from build123d import *

# Parameters (mm, degrees)
F0_R     = 10.002614
F0_W     = 8.257874
F0_H     = 10.88538
F0_R_2   = 19.05
F1_DEPTH = 3.175


with BuildPart() as f1:
    # F0 (on Front) → F1 (new body)
    with BuildSketch(Plane.XZ):
        with BuildLine():
            ThreePointArc((75.042351, -13.231991), (75.910036, -6.641268), (76.2, 0))
            ThreePointArc((76.2, 0), (76.134965, 3.14755), (75.939972, 6.289727))
            ThreePointArc((75.939972, 6.289727), (75.570922, 9.771172), (75.042351, 13.231991))
            ThreePointArc((75.042351, 13.231991), (72.726083, 22.745479), (69.209018, 31.88341))
            ThreePointArc((69.209018, 31.88341), (67.6715, 35.028675), (65.991136, 38.1))
            ThreePointArc((65.991136, 38.1), (60.560752, 46.247544), (54.130435, 53.631483))
            ThreePointArc((54.130435, 53.631483), (51.609896, 56.061204), (48.980416, 58.372587))
            ThreePointArc((48.980416, 58.372587), (41.0909, 64.171473), (32.522923, 68.910808))
            ThreePointArc((32.522923, 68.910808), (29.323378, 70.331924), (26.061935, 71.604578))
            ThreePointArc((26.061935, 71.604578), (16.664879, 74.355375), (6.992666, 75.878473))
            ThreePointArc((6.992666, 75.878473), (3.500027, 76.119576), (0, 76.2))
            ThreePointArc((0, 76.2), (-9.771172, 75.570922), (-19.381009, 73.694074))
            ThreePointArc((-19.381009, 73.694074), (-22.745479, 72.726083), (-26.061935, 71.604578))
            ThreePointArc((-26.061935, 71.604578), (-35.028675, 67.6715), (-43.417049, 62.621082))
            ThreePointArc((-43.417049, 62.621082), (-46.247544, 60.560752), (-48.980416, 58.372587))
            ThreePointArc((-48.980416, 58.372587), (-56.061204, 51.609896), (-62.216352, 43.995063))
            ThreePointArc((-62.216352, 43.995063), (-64.171473, 41.0909), (-65.991136, 38.1))
            ThreePointArc((-65.991136, 38.1), (-70.331924, 29.323378), (-73.511444, 20.06259))
            ThreePointArc((-73.511444, 20.06259), (-74.355375, 16.664879), (-75.042351, 13.231991))
            ThreePointArc((-75.042351, 13.231991), (-76.119576, 3.500027), (-75.939972, -6.289727))
            ThreePointArc((-75.939972, -6.289727), (-75.570922, -9.771172), (-75.042351, -13.231991))
            ThreePointArc((-75.042351, -13.231991), (-72.726083, -22.745479), (-69.209018, -31.88341))
            ThreePointArc((-69.209018, -31.88341), (-67.6715, -35.028675), (-65.991136, -38.1))
            ThreePointArc((-65.991136, -38.1), (-60.560752, -46.247544), (-54.130435, -53.631483))
            ThreePointArc((-54.130435, -53.631483), (-51.609896, -56.061204), (-48.980416, -58.372587))
            ThreePointArc((-48.980416, -58.372587), (-41.0909, -64.171473), (-32.522923, -68.910808))
            ThreePointArc((-32.522923, -68.910808), (-29.323378, -70.331924), (-26.061935, -71.604578))
            ThreePointArc((-26.061935, -71.604578), (-16.664879, -74.355375), (-6.992666, -75.878473))
            ThreePointArc((-6.992666, -75.878473), (-3.500027, -76.119576), (0, -76.2))
            ThreePointArc((0, -76.2), (9.771172, -75.570922), (19.381009, -73.694074))
            ThreePointArc((19.381009, -73.694074), (22.745479, -72.726083), (26.061935, -71.604578))
            ThreePointArc((26.061935, -71.604578), (35.028675, -67.6715), (43.417049, -62.621082))
            ThreePointArc((43.417049, -62.621082), (46.247544, -60.560752), (48.980416, -58.372587))
            ThreePointArc((48.980416, -58.372587), (56.061204, -51.609896), (62.216352, -43.995063))
            ThreePointArc((62.216352, -43.995063), (64.171473, -41.0909), (65.991136, -38.1))
            ThreePointArc((65.991136, -38.1), (70.331924, -29.323378), (73.511444, -20.06259))
            ThreePointArc((73.511444, -20.06259), (74.355375, -16.664879), (75.042351, -13.231991))
        make_face()
        with Locations((-32.771484, -33.103804)):
            Circle(F0_R, mode=Mode.SUBTRACT)
        with Locations((1.650614, -45.994491)):
            Circle(F0_R, mode=Mode.SUBTRACT)
        with Locations((35.105805, -30.769484)):
            Circle(F0_R, mode=Mode.SUBTRACT)
        with Locations((-47.996491, 0.351386)):
            Circle(F0_R, mode=Mode.SUBTRACT)
        with Locations((-25.4, 0)):
            Rectangle(F0_W, F0_H, mode=Mode.SUBTRACT)
        with Locations((-35.105805, 34.773484)):
            Circle(F0_R, mode=Mode.SUBTRACT)
        with Locations((-1.650614, 49.998491)):
            Circle(F0_R, mode=Mode.SUBTRACT)
        Circle(F0_R_2, mode=Mode.SUBTRACT)
        with Locations((25.4, 0)):
            Rectangle(F0_W, F0_H, mode=Mode.SUBTRACT)
        with Locations((32.771484, 37.107805)):
            Circle(F0_R, mode=Mode.SUBTRACT)
        with Locations((47.996491, 3.652614)):
            Circle(F0_R, mode=Mode.SUBTRACT)
        with BuildLine():
            ThreePointArc((75.042351, 13.231991), (75.570922, 9.771172), (75.939972, 6.289727))
            Line((75.939972, 6.289727), (93.646024, 16.512321))
            Line((93.646024, 16.512321), (75.042351, 13.231991))
        make_face()
        with BuildLine():
            Line((93.646024, -16.512321), (75.042351, -13.231991))
            ThreePointArc((75.042351, -13.231991), (74.355375, -16.664879), (73.511444, -20.06259))
            Line((73.511444, -20.06259), (93.646024, -16.512321))
        make_face()
        with BuildLine():
            ThreePointArc((65.991136, 38.1), (67.6715, 35.028675), (69.209018, 31.88341))
            Line((69.209018, 31.88341), (82.350931, 47.545332))
            Line((82.350931, 47.545332), (65.991136, 38.1))
        make_face()
        with BuildLine():
            Line((82.350931, -47.545332), (65.991136, -38.1))
            ThreePointArc((65.991136, -38.1), (64.171473, -41.0909), (62.216352, -43.995063))
            Line((62.216352, -43.995063), (82.350931, -47.545332))
        make_face()
        with BuildLine():
            ThreePointArc((48.980416, 58.372587), (51.609896, 56.061204), (54.130435, 53.631483))
            Line((54.130435, 53.631483), (61.123101, 72.843675))
            Line((61.123101, 72.843675), (48.980416, 58.372587))
        make_face()
        with BuildLine():
            Line((61.123101, -72.843675), (48.980416, -58.372587))
            ThreePointArc((48.980416, -58.372587), (46.247544, -60.560752), (43.417049, -62.621082))
            Line((43.417049, -62.621082), (61.123101, -72.843675))
        make_face()
        with BuildLine():
            ThreePointArc((26.061935, 71.604578), (29.323378, 70.331924), (32.522923, 68.910808))
            Line((32.522923, 68.910808), (32.522923, 89.355996))
            Line((32.522923, 89.355996), (26.061935, 71.604578))
        make_face()
        with BuildLine():
            Line((32.522923, -89.355996), (26.061935, -71.604578))
            ThreePointArc((26.061935, -71.604578), (22.745479, -72.726083), (19.381009, -73.694074))
            Line((19.381009, -73.694074), (32.522923, -89.355996))
        make_face()
        with BuildLine():
            ThreePointArc((0, 76.2), (3.500027, 76.119576), (6.992666, 75.878473))
            Line((6.992666, 75.878473), (0, 95.090665))
            Line((0, 95.090665), (0, 76.2))
        make_face()
        with BuildLine():
            Line((0, -95.090665), (0, -76.2))
            ThreePointArc((0, -76.2), (-3.500027, -76.119576), (-6.992666, -75.878473))
            Line((-6.992666, -75.878473), (0, -95.090665))
        make_face()
        with BuildLine():
            ThreePointArc((-26.061935, 71.604578), (-22.745479, 72.726083), (-19.381009, 73.694074))
            Line((-19.381009, 73.694074), (-32.522923, 89.355996))
            Line((-32.522923, 89.355996), (-26.061935, 71.604578))
        make_face()
        with BuildLine():
            Line((-32.522923, -89.355996), (-26.061935, -71.604578))
            ThreePointArc((-26.061935, -71.604578), (-29.323378, -70.331924), (-32.522923, -68.910808))
            Line((-32.522923, -68.910808), (-32.522923, -89.355996))
        make_face()
        with BuildLine():
            ThreePointArc((-48.980416, 58.372587), (-46.247544, 60.560752), (-43.417049, 62.621082))
            Line((-43.417049, 62.621082), (-61.123101, 72.843675))
            Line((-61.123101, 72.843675), (-48.980416, 58.372587))
        make_face()
        with BuildLine():
            Line((-61.123101, -72.843675), (-48.980416, -58.372587))
            ThreePointArc((-48.980416, -58.372587), (-51.609896, -56.061204), (-54.130435, -53.631483))
            Line((-54.130435, -53.631483), (-61.123101, -72.843675))
        make_face()
        with BuildLine():
            ThreePointArc((-65.991136, 38.1), (-64.171473, 41.0909), (-62.216352, 43.995063))
            Line((-62.216352, 43.995063), (-82.350931, 47.545332))
            Line((-82.350931, 47.545332), (-65.991136, 38.1))
        make_face()
        with BuildLine():
            Line((-82.350931, -47.545332), (-65.991136, -38.1))
            ThreePointArc((-65.991136, -38.1), (-67.6715, -35.028675), (-69.209018, -31.88341))
            Line((-69.209018, -31.88341), (-82.350931, -47.545332))
        make_face()
        with BuildLine():
            ThreePointArc((-75.042351, 13.231991), (-74.355375, 16.664879), (-73.511444, 20.06259))
            Line((-73.511444, 20.06259), (-93.646024, 16.512321))
            Line((-93.646024, 16.512321), (-75.042351, 13.231991))
        make_face()
        with BuildLine():
            Line((-93.646024, -16.512321), (-75.042351, -13.231991))
            ThreePointArc((-75.042351, -13.231991), (-75.570922, -9.771172), (-75.939972, -6.289727))
            Line((-75.939972, -6.289727), (-93.646024, -16.512321))
        make_face()
    extrude(amount=F1_DEPTH)


solid = f1.part
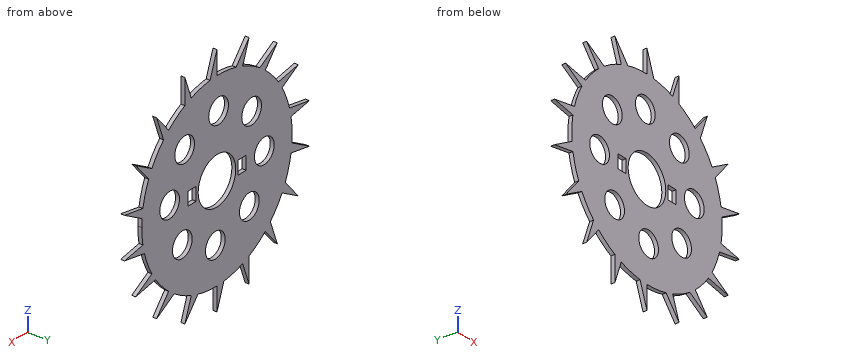
Read the model definition and answer for the solid it produces. Units are mm, in the model's axes. Coordinates: 2 decimals unless noted, no trailing zeros. Answer in a Markdown table with one row per item.
Item 1: Straight lines are drawn through the part: line 1 along X through (y, z) = (-0.55, -33.5); line 2 along Z through (x, y) = (8.5, -2.75); line 3 along X through (y, z) = (-2.7, 36). For each, find the intervals that lie inside material, in ascending order. Write a range as [from, to].
Returned:
| item | result |
|---|---|
| line 1 | x = [-70.57, -42.77], [-22.78, 25.48], [44.73, 68.44] |
| line 2 | z = [-75.72, -53.28], [-38.7, -17.05], [17.05, 75.72] |
| line 3 | x = [-67.16, -45.03], [-25.18, 22.83], [42.71, 72.66] |
Item 2: Each of these flat-tipped pins is pushed along its axis until it touches: P1, Ø1, axis at y = -1, z = -89, coming from the +X side; P2, Ø1, axis at y = -1, z = -1.5, coming from the +X side; P3, Ø1, axis at y = -2, z = 83.5, coming from the -X side. Where does it stop, or does it pass through?
Returned:
| item | result |
|---|---|
| P1 | stops at x = 32.52 |
| P2 | stops at x = 76.19 |
| P3 | stops at x = -30.57 |
Item 3: A cutting plane is placed at A-A on y = -1.2. Give the number of separate pieces and of enclosed holes in the cut face, plus the area to 3 significant figures.
Returned:
| item | result |
|---|---|
| separate pieces | 1 |
| enclosed holes | 11 |
| area | 15,600 mm^2 |
